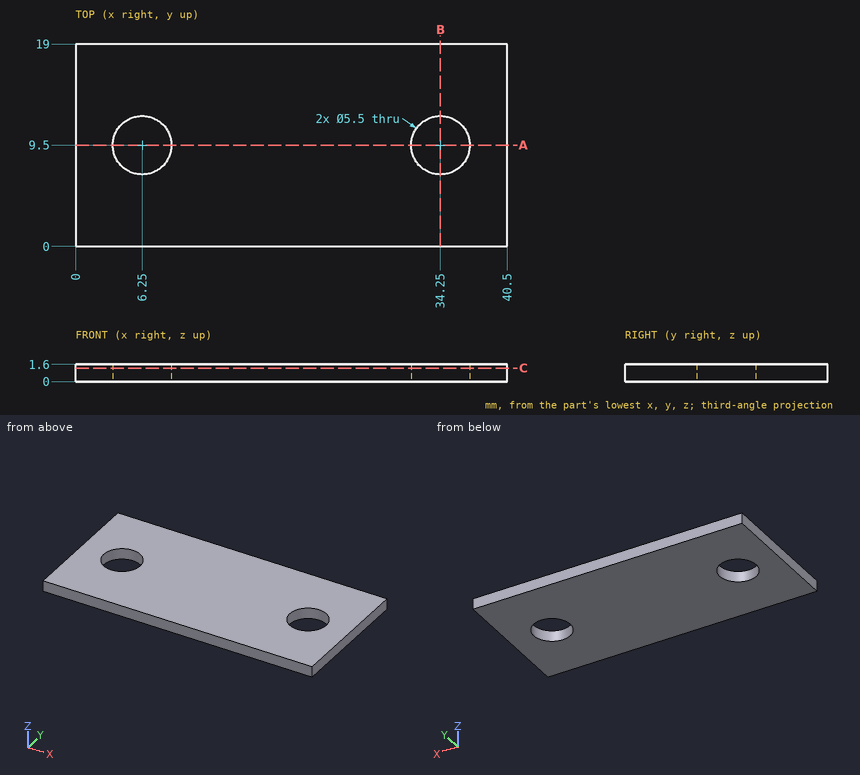
Can you work these out from the drawing? Everything is in mm from the part's minimum corner. Give positions to 0.01 mm unless a question says otherwise; leave off trailing zeros. Order: outer loops, then holes, each group sorted by start corner. A loop starts at its lowest first (then second) coordinate and runs counter-clockwise, first axis right, second up.
1. I need wall thicknesses on L1, parallel to X at y = 9.5, z = 0.6; L2, parallel to Y at x = 34.25, z = 1.2; L3, parallel to X at y = 8.5, z = 0.6. Which ranges of each line are inside material? Lowest first, please.
2. Suppose I cut it at C-C (z = 1.25). List the corners of the cut face in (x, y) for me, plus the area to 3 significant figures.
3. Suppose I cut it at A-A (y = 9.5). List the corners of the cut face in (x, z) for me.
4. Suppose I cut it at B-B (x = 34.25). List the corners of the cut face in (y, z) for me, plus the area to 3 significant figures.
Solved:
1. L1: x = 0 to 3.5, 9 to 31.5, 37 to 40.5
1. L2: y = 0 to 6.75, 12.25 to 19
1. L3: x = 0 to 3.69, 8.81 to 31.69, 36.81 to 40.5
2. outline: (0, 0) - (40.5, 0) - (40.5, 19) - (0, 19) - close; hole circle Ø5.5 at (6.25, 9.5); hole circle Ø5.5 at (34.25, 9.5)
2. area: 722 mm2
3. outline: (0, 0) - (3.5, 0) - (3.5, 1.6) - (0, 1.6) - close; (9, 0) - (31.5, 0) - (31.5, 1.6) - (9, 1.6) - close; (37, 0) - (40.5, 0) - (40.5, 1.6) - (37, 1.6) - close
4. outline: (0, 0) - (6.75, 0) - (6.75, 1.6) - (0, 1.6) - close; (12.25, 0) - (19, 0) - (19, 1.6) - (12.25, 1.6) - close
4. area: 21.6 mm2
